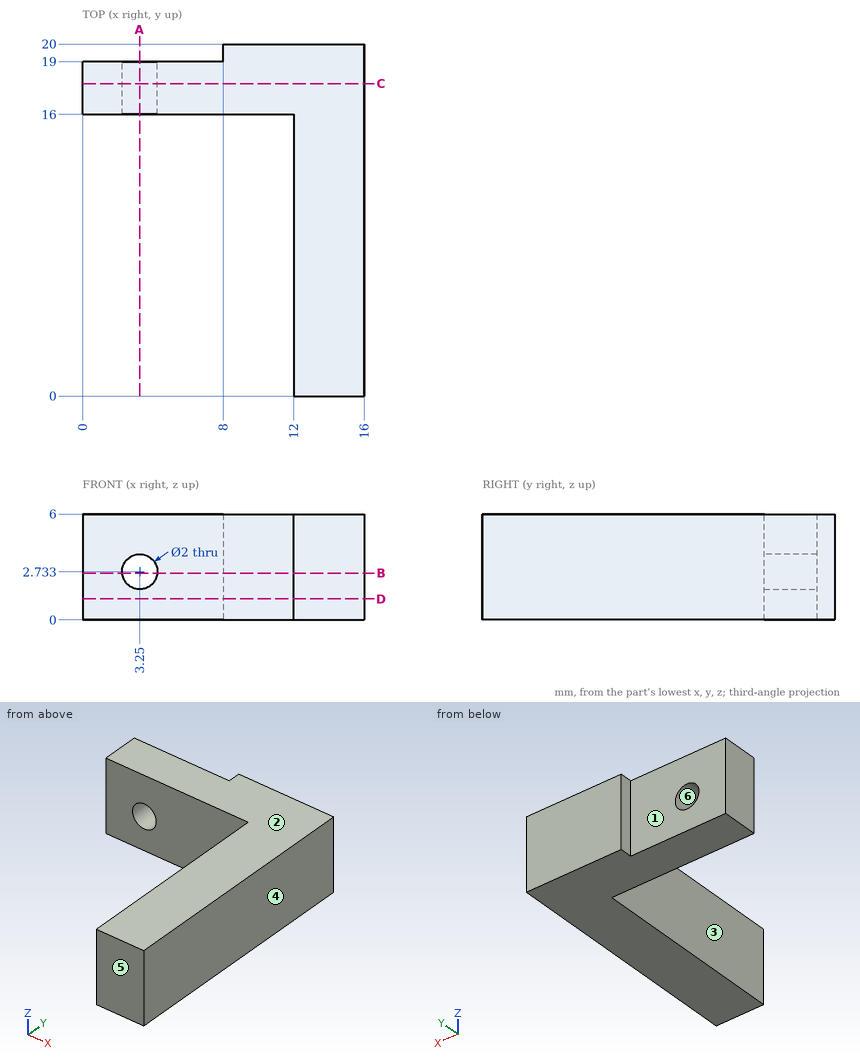
Geometry: see drawing. Coordinates: mm, zero at the bounding-box minimum. A direction names the side the tool comes from. Give positions to 0.01 mm unless a question says otherwise; leave off trailing zeros. Loops run counter-clockwise (first coordinate to the right, second up) from the corner with the lowest first, then second, coordinate; pieces in that order, holes last. Notation, with made-up numbers: (-24.75, -13) - (-5.75, -13) arc R29 ccw to (-5.75, 19) - close; hole circle Ø8 at (20.25, 60). An arc over 180 degrees is marked (long way). One line per question, with ' | ' between items. Start each with the question number.
(1) Section query A-A on x = 3.25. Return loops of the section in (y, z), then the cut area to 3 significant figures.
(2) Pull-direction query (X, two-part tool) for the marked faces 4, 5 and 6; classes: released by +X, released by -X, zero draft, split by the parting line, or undercut.
(3) Reachability of the marked faces 1, 2 and 3 from +Z, -Z, +X, -X, +Y, -Y: full face, straight path, thin tool, end or side. Return the list, or none.
(4) Ray query, line 1 (X direction, y = 9, z = 1.7); line 2 (Y direction, x = 1.75, z = 4.5); line 3 (Y direction, x = 9.5, z = 4.3). Return the intervals inside material, ascending. Write a range as from..to.
(5) Section query B-B on z = 2.65. Return loops of the section in (x, y), then the cut area to 3 significant figures.
(6) Section query C-C on y = 17.75. Return loops of the section in (x, z).
(7) Section query D-D on z = 1.2. Return loops of the section in (x, y).
(8) Contact query for flat-ended pins moving along their axis: pin 1 (2 mm diameter, centred on x = 3, y = 14, fed in from +Z); pin 2 (1.1 mm diameter, centred on y = 19.5, z = 2.5, fed in from -X); pin 3 (1.5 mm diameter, centred on x = 3.5, z = 5, fed in from +Y); pin 4 (1.8 mm diameter, centred on x = 3.5, z = 2, fed in from -Y). Output: stop coordinate, or through.
The answers:
1) outline: (16, 0) - (19, 0) - (19, 1.73) - (16, 1.73) - close; (16, 3.73) - (19, 3.73) - (19, 6) - (16, 6) - close | area: 12.0 mm2
2) face 4: released by +X | face 5: zero draft | face 6: undercut
3) face 1: +Z, -Z, -X, +Y | face 2: +Z, +X, -X, +Y, -Y | face 3: +Z, -Z, -X, -Y
4) line 1: 12..16 | line 2: 16..19 | line 3: 16..20
5) outline: (0, 16) - (2.25, 16) - (2.25, 19) - (0, 19) - close; (4.25, 16) - (12, 16) - (12, 0) - (16, 0) - (16, 20) - (8, 20) - (8, 19) - (4.25, 19) - close | area: 114 mm2
6) outline: (0, 0) - (16, 0) - (16, 6) - (0, 6) - close; hole circle Ø2 at (3.25, 2.73)
7) outline: (0, 16) - (12, 16) - (12, 0) - (16, 0) - (16, 20) - (8, 20) - (8, 19) - (0, 19) - close
8) pin 1: through | pin 2: x = 0 | pin 3: y = 19 | pin 4: y = 16
